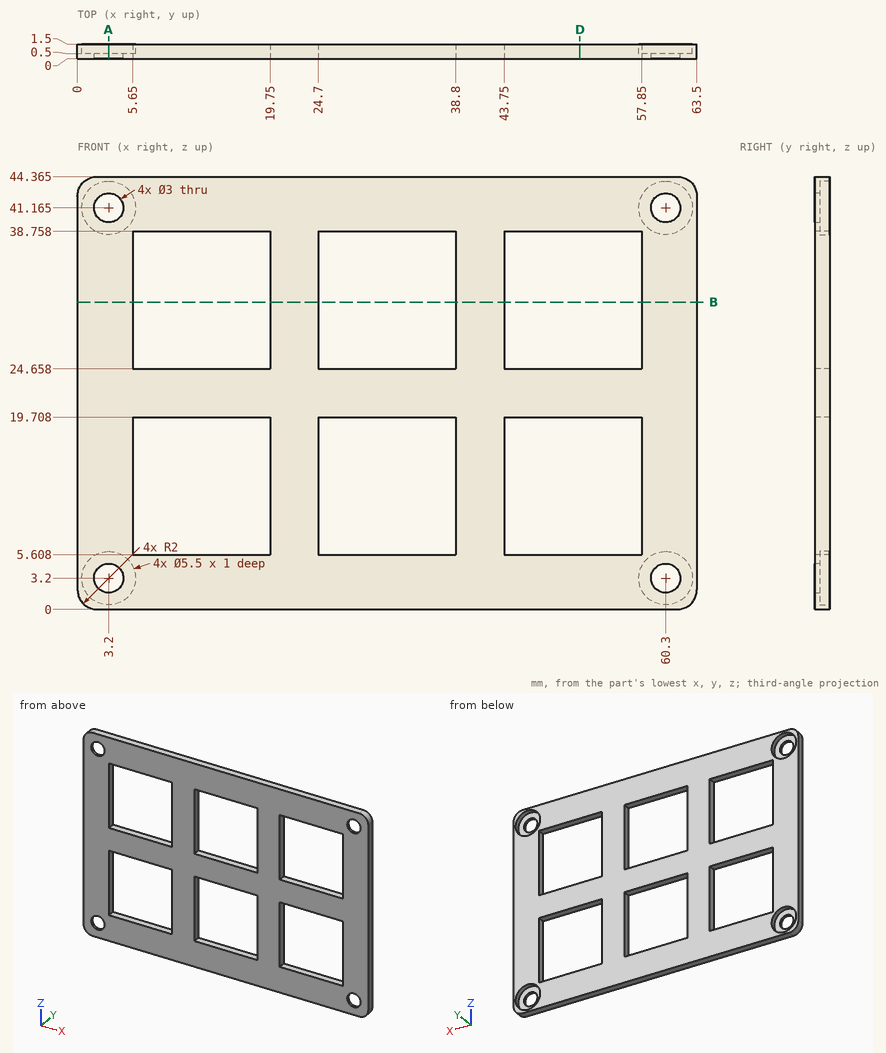
Answer from the drawing. Dimensions are ordinates in mm from the lowest x, y and z of the part. Round coordinates to 2 decimals unless told otherwise and drop trailing zeros. Loops run counter-clockwise (first coordinate to the right, second up) from the corner with the lowest first, then second, coordinate; pieces in that order, holes last.
Q1. Section B-B on z = 31.5 is taken. Write down the section's boundary in (x, y).
Q2. Section D-D on x = 51.5 is taken. Write down the section's boundary in (y, z) (1 decimal).
Q3. Section A-A on x = 3.2 is taken. Give the number of separate pieces and of enclosed holes in the cut face.
Q4. Consider probe 1 along X at (y, z) = (1.4, 36); probe 2 along Z at (x, y) = (38, 1.15) (1 decimal); probe 3 along X at (y, z) = (0.25, 3.2). Determine where each line is inside the solid, lowest interval first.
Q5. This flat-tipped pin is pushed along its axis until it touches: pin 1 (4.5 mm diameter, centred on x = 60.5, z = 3.5, fed in from +Y). Where does it stop, or does it pass through?
Output:
1. outline: (0, 0) - (5.65, 0) - (5.65, 1.5) - (0, 1.5) - close; (19.75, 0) - (24.7, 0) - (24.7, 1.5) - (19.75, 1.5) - close; (38.8, 0) - (43.75, 0) - (43.75, 1.5) - (38.8, 1.5) - close; (57.85, 0) - (63.5, 0) - (63.5, 1.5) - (57.85, 1.5) - close
2. outline: (0, 0) - (1.5, 0) - (1.5, 5.6) - (0, 5.6) - close; (0, 19.7) - (1.5, 19.7) - (1.5, 24.7) - (0, 24.7) - close; (0, 38.8) - (1.5, 38.8) - (1.5, 44.4) - (0, 44.4) - close
3. separate pieces: 3
3. enclosed holes: 0
4. probe 1: x = 0 to 5.65, 19.75 to 24.7, 38.8 to 43.75, 57.85 to 63.5
4. probe 2: z = 0 to 5.6, 19.7 to 24.7, 38.8 to 44.4
4. probe 3: x = 0 to 1.7, 4.7 to 58.8, 61.8 to 63.5
5. pin 1: stops at y = 0.5
